Design review of the part built by this model. Coordinates are the model's own, in mm. A direction names the side the tool comes from. Coordinates: 2 decimals unless noted, no trailing zeros. Loops run counter-clockwise (first coordinate to the right, second up) from the corner with the lowest first, then second, coordinate; pieces in that order, holes last. Notation, with made-up numbers: (3.25, -6) - (10.25, -6) arc R32 cw to (10.25, 32) - close; hole circle Ø11 at (50, 65.25). An arc over 180 degrees is marked (long way). Answer in a Markdown table with one row per item. Add a question column.
(1) We need section C-C, the plane y = -5.5. Write out the cut boundary in (x, z).
(2) For faces 1 (the face through (-1.5, -4.68, 0.07)), 2 (the face through (-0.54, -9.99, -2.44)), list the 3-axis set-ups (+Z, -Z, +X, -X, +Y, -Y) from which the entire face can be reached by the end or side of a thin tool; tool diameter is ignored.
(3) To check wall thickness, follow L1, parallel to X at y = -5.25, z = 0.05; L2, parallel to Y at x = -1.4, z = -1; L3, parallel to Y at x = -1, z = -0.95. State the ranges of each line that lie inside material, in increasing order. Write a range as [from, to].
(4) The part is to be moulded in two halves that separate along Y. For faces 3 (the face through (0, 1, 0)), 4 (the face through (0.27, 0.25, -1.22)), 5 (the face through (0, -10.5, 0)), 6 (the face through (1.5, 0.75, 0.07)), say which applies: released by +Y, released by -Y, zero draft, split by the parting line, or undercut.
(5) Clearance check with flat-ended pins moving along their axes: pin 1 (1.5 mm diameter, centred on y = -3, z = 0, fed in from -X); pin 2 (2 mm diameter, centred on x = -2, y = -1, fed in from +Z). State where each tip first meets the part, or that it passes through.
(6) We need section D-D, the plane z = 2. Write out the cut boundary in (x, y).
(7) We need section A-A, the plane z = 0. Write out the cut boundary in (x, y).
(8) We need section B-B, the plane x = 0.35. Write out the cut boundary in (y, z).
from build123d import *

# Parameters (mm, degrees)
F0_R     = 1.5
F1_DEPTH = 9.5
F2_R     = 2.5
F3_DEPTH = 1
F4_R     = 1.25
F5_DEPTH = 0.5
F6_R     = 1.5
F7_DEPTH = 0.5


with BuildPart() as f1:
    # F0 (on Front) → F1 (new body)
    with BuildSketch(Plane.XZ):
        Circle(F0_R)
    extrude(amount=F1_DEPTH)

    # F2 (on face) → F3 (join)
    with BuildSketch(Plane.XZ.offset(9.5)):
        Circle(F2_R)
    extrude(amount=F3_DEPTH)

    # F4 (on face) → F5 (join)
    with BuildSketch(Plane(origin=(0, 0, 0), x_dir=(-1, 0, 0), z_dir=(0, 1, 0))):
        Circle(F4_R)
    extrude(amount=F5_DEPTH)

    # F6 (on face) → F7 (join)
    with BuildSketch(Plane(origin=(0, 0.5, 0), x_dir=(-1, 0, 0), z_dir=(0, 1, 0))):
        Circle(F6_R)
    extrude(amount=F7_DEPTH)


solid = f1.part
Responses:
| question | item | result |
|---|---|---|
| 1 | outline | circle Ø3 at (0, 0) |
| 2 | face 1 | +Y |
| 2 | face 2 | +Y, -Y |
| 3 | L1 | x = [-1.5, 1.5] |
| 3 | L2 | y = [-10.5, -9.5] |
| 3 | L3 | y = [-10.5, 0], [0.5, 1] |
| 4 | face 3 | released by +Y |
| 4 | face 4 | undercut |
| 4 | face 5 | released by -Y |
| 4 | face 6 | zero draft |
| 5 | pin 1 | stops at x = -1.5 |
| 5 | pin 2 | stops at z = 1.12 |
| 6 | outline | (-1.5, -10.5) - (1.5, -10.5) - (1.5, -9.5) - (-1.5, -9.5) - close |
| 7 | outline | (-2.5, -10.5) - (2.5, -10.5) - (2.5, -9.5) - (1.5, -9.5) - (1.5, 0) - (1.25, 0) - (1.25, 0.5) - (1.5, 0.5) - (1.5, 1) - (-1.5, 1) - (-1.5, 0.5) - (-1.25, 0.5) - (-1.25, 0) - (-1.5, 0) - (-1.5, -9.5) - (-2.5, -9.5) - close |
| 8 | outline | (-10.5, -2.48) - (-9.5, -2.48) - (-9.5, -1.46) - (0, -1.46) - (0, -1.2) - (0.5, -1.2) - (0.5, -1.46) - (1, -1.46) - (1, 1.46) - (0.5, 1.46) - (0.5, 1.2) - (0, 1.2) - (0, 1.46) - (-9.5, 1.46) - (-9.5, 2.48) - (-10.5, 2.48) - close |
